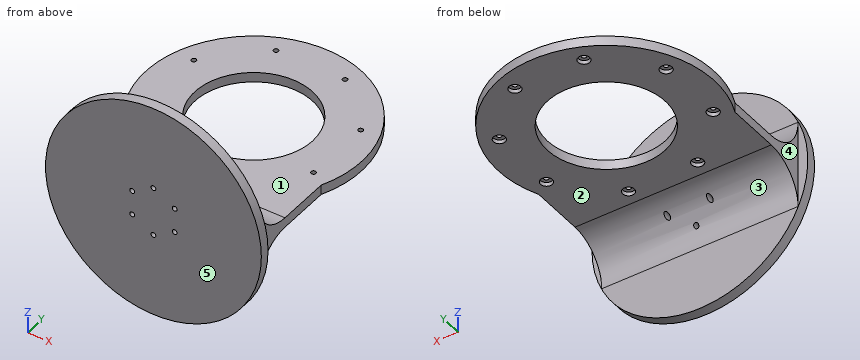
Autodesk Inventor part; units mm, degrees
ref_plane "YZ Plane" through (0, 0, 0) normal (1, 0, 0) x (0, 1, 0)
ref_plane "XZ Plane" through (0, 0, 0) normal (0, 1, 0) x (-1, 0, 0)
ref_plane "XY Plane" through (0, 0, 0) normal (0, 0, 1) x (1, 0, 0)
sketch "スケッチ1" plane through (0, 0, 0) normal (0, 0, 1) x (1, 0, 0)
  circle A0 centre (0, 0) radius 48.5
  circle A1 centre (0, 0) radius 30
  line L0 (-50, 50) -> (50, 50)
  line L1 (50, 50) -> (50, -50)
  line L2 (50, -50) -> (-50, -50)
  line L3 (-50, -50) -> (-50, 50)
  line L4 (-50, -50) -> (50, -50)
  line L5 (50, -50) -> (50, -70)
  line L6 (50, -70) -> (-50, -70)
  line L7 (-50, -70) -> (-50, -50)
  circle A2 centre (0, 0) radius 55
  point P0 (-50, -60)
  point P1 (-50, -22.9129)
  point P2 (50, -22.9129)
  dimension "d0" = 97
  dimension "d3" = 50
  dimension "d4" = 50
  dimension "d5" = 50
  dimension "d6" = 50
  dimension "d126" = 20
  dimension "d127" = 100
  dimension "d128" = 110
  dimension "d129" = 60
extrude "押し出し1" add sketch "スケッチ1" along normal blind 5 contours A0 | A1 | A2 L0 | L0 A2 L1 L2 L3 | L3 A2 | A2 L2 L3 | A2 L1 | L2 A2 L5 L6 L7 | L2 A2 | L1 L2 A2
sketch "スケッチ2" plane through (0, 0, 5) normal (0, 0, 1) x (1, 0, 0)
  circle A0 centre (0, 0) radius 46
  line L0 (0, 0) -> (0, 64.6511)
  line L1 (0, 0) -> (-25.9524, 62.6547)
  line L2 (-50, -22.9129) -> (-50, -70)
  point P0 (-17.6034, 42.4985)
  point P1 (-42.4985, 17.6034)
  point P2 (-42.4985, -17.6034)
  point P3 (-17.6034, -42.4985)
  point P4 (17.6034, -42.4985)
  point P5 (42.4985, -17.6034)
  point P6 (42.4985, 17.6034)
  point P7 (17.6034, 42.4985)
  point P8 (-50, 50)
  point P9 (-50, -50)
  dimension "d7" = 92
  dimension "d8" = 22.5
  dimension "d11" = 360
  dimension "d76" = 50
hole "穴1" at (-17.6034, 42.4985, 5) at (-42.4985, 17.6034, 5) at (-42.4985, -17.6034, 5) at (-17.6034, -42.4985, 5) at (17.6034, -42.4985, 5) at (42.4985, -17.6034, 5) at (42.4985, 17.6034, 5) at (17.6034, 42.4985, 5) direction (0, 0, -1) diameter 2.459 end through all
sketch "スケッチ3" plane through (0, 0, 5) normal (0, 0, 1) x (1, 0, 0)
  circle A0 centre (0, 0) radius 30
  dimension "d20" = 60
extrude "押し出し2" cut sketch "スケッチ3" against normal blind 5
sketch "スケッチ16" plane through (0, 0, 0) normal (0, 0, -1) x (-1, 0, 0)
  circle A0 centre (17.6034, 42.4985) radius 1.2295
  circle A1 centre (0, 0) radius 46
  circle A2 centre (17.6034, 42.4985) radius 3
  circle A3 centre (-17.6034, 42.4985) radius 3
  circle A4 centre (-42.4985, 17.6034) radius 3
  circle A5 centre (-42.4985, -17.6034) radius 3
  circle A6 centre (-17.6034, -42.4985) radius 3
  circle A7 centre (17.6034, -42.4985) radius 3
  circle A8 centre (42.4985, -17.6034) radius 3
  circle A9 centre (42.4985, 17.6034) radius 3
  point P0 (18.7653, 42.0962)
  point P1 (16.4975, 43.0356)
  dimension "d113" = 6
  dimension "d116" = 360
extrude "押し出し12" cut sketch "スケッチ16" against normal blind 2 contours A0 A1 | A0 A1 A2 | A1 A0 | A0 A1 A2 | A3 A1 | A1 A3 | A9 A1 | A1 A9 | A4 A1 | A1 A4 | A8 A1 | A1 A8 | A5 A1 | A1 A5 | A7 A1 | A1 A7 | A6 A1 | A1 A6
sketch "スケッチ19" plane through (-50, -70, 0) normal (0, -1, 0) x (1, 0, 0)
  line L0 (0, 5) -> (100, 5)
  line L1 (0, 5) -> (100, 5)
  line L2 (100, 5) -> (100, -47.5)
  line L3 (100, -47.5) -> (0, -47.5)
  line L4 (0, -47.5) -> (0, 5)
  line L5 (0, -47.5) -> (100, -47.5)
  line L6 (100, -47.5) -> (100, 52.5)
  line L7 (100, 52.5) -> (0, 52.5)
  line L8 (0, 52.5) -> (0, -47.5)
  circle A0 centre (50, 2.5) radius 55
  point P0 (50, 0)
  dimension "d130" = 100
  dimension "d131" = 47.5
  dimension "d132" = 100
  dimension "d136" = 110
  dimension "d137" = 50
  dimension "d138" = 50
extrude "押し出し14" add sketch "スケッチ19" along normal blind 5 contours L8 A0 L7 L6 L0 | L0 L2 A0 L3 L4 | L4 A0 L8 | L6 A0 L2 | L3 A0 | A0 L7
fillet "フィレット6" radius 20 2 edges at (0, -70, 5) (0, -70, 0)
sketch "スケッチ20" plane through (0, -75, 2.5) normal (0, -1, 0) x (1, 0, 0)
  circle A0 centre (0, 0) radius 12.5
  line L0 (-10.8253, -6.25) -> (0, 0)
  line L1 (0, 0) -> (-14.9018, 0)
  point P0 (0, -2.5)
  point P1 (0, -12.5)
  point P2 (10.8253, -6.25)
  point P3 (10.8253, 6.25)
  point P4 (0, 12.5)
  point P5 (-10.8253, 6.25)
  dimension "d139" = 25
  dimension "d140" = 30
  dimension "d143" = 360
hole "穴5" at (-10.8253, -75, -3.75) at (0, -75, -10) at (10.8253, -75, -3.75) at (10.8253, -75, 8.75) at (0, -75, 15) at (-10.8253, -75, 8.75) direction (0, 1, 0) diameter 2.459 end through all
properties part number "legparts_07(five)"
The model under review builds one solid part; all positions refer to its coordinate system, in mm. Face numbers are marked on the shaded views. A direction names the side the tool comes from. Give positions to 0.01 mm unless a question says otherwise; leave off trailing zeros. Write each loop counter-clockwise with the first axis right and the second up, starting at its lowest first coordinate (ties: lowest second). Pieces come first, ordered by that corner, then holes. Notation, with made-up numbers: M 23.5,66.5 L 36.5,66.5 A28 ccw 36.5,102.5 Z; hole C 47.25,85.5 d11. An arc over 180 degrees is marked long. Answer in a Markdown table with one row per item.
Item 1: Add section B-B on x = 35. Give the boundary of the cut face in (y, z), plus the area to 3 significant figures.
Check sheet entries:
| item | result |
|---|---|
| outline | M -75,-39.93 L -70,-39.93 L -70,-20 A20 cw -50,0 L 42.43,0 L 42.43,5 L -50,5 A20 cw -70,25 L -70,44.93 L -75,44.93 Z |
| area | 1,160 mm2 |
Item 2: For line 1 along X through (y, z) = (-68, 8); line 2 along Z through (x, y) = (19.5, -27.5); line 3 along Y through (x, z) = (-27, -24.5), list the stretches that pass through material, from the lowest coordinate up.
Check sheet entries:
| item | result |
|---|---|
| line 1 | -50 to -11.8, -9.85 to 9.85, 11.8 to 50 |
| line 2 | 0 to 5 |
| line 3 | -75 to -70 |
Item 3: Draft analysis for pull direction Y (two halves, no side actions). For the marked faces 3, 4 and 5, state which applies: +Y half, -Y half, draft (parallel to the pull), parting line (faces both ways), or undercut.
Check sheet entries:
| item | result |
|---|---|
| face 3 | +Y half |
| face 4 | undercut |
| face 5 | -Y half |
Item 4: For P1, Ø5, axis at x = -17, y = -41.5, coming from the -Z side; P2, Ø2, axis at x = -10.83, z = 8.75, coming from the +Y side; P3, Ø12, axis at x = -14.5, z = 37.5, coming from the +Y side; P4, Ø3, axis at x = 0, z = -10, coming from the -Y side, all flat-tipped, find the tip position at first contact; note any pin that passes through.
Check sheet entries:
| item | result |
|---|---|
| P1 | z = 0 |
| P2 | through |
| P3 | y = -70 |
| P4 | y = -75 |
Item 5: Add section D-D on y = -61.5. Give the boundary of the cut face in (x, z), plus the area to 3 significant figures.
Check sheet entries:
| item | result |
|---|---|
| outline | M -50,-3.64 L -12.05,-3.64 A1.23 cw -9.6,-3.64 L 9.6,-3.64 A1.23 cw 12.05,-3.64 L 50,-3.64 L 50,8.64 L 12.05,8.64 A1.23 cw 9.6,8.64 L -9.6,8.64 A1.23 cw -12.05,8.64 L -50,8.64 Z |
| area | 1,220 mm2 |
Item 6: Add section C-C on x = 7.5. Give the boundary of the cut face in (y, z), plus the area to 3 significant figures.
Check sheet entries:
| item | result |
|---|---|
| outline | M -75,-51.99 L -70,-51.99 L -70,-20 A20 cw -50,0 L -29.05,0 L -29.05,5 L -50,5 A20 cw -70,25 L -70,56.99 L -75,56.99 Z; M 29.05,0 L 54.49,0 L 54.49,5 L 29.05,5 Z |
| area | 1,050 mm2 |
Item 7: Tool access review of the marked faces 1 and 2: name each direction out of +Z, -Z, +X, -X, +Y, -Y from which nothing blocks a thin tool from reaching the whole face with its end or side.
Check sheet entries:
| item | result |
|---|---|
| face 1 | +Z, +X, -X, +Y |
| face 2 | -Z, +X, -X, +Y |
Item 8: Add section A-A on y = 0. Give the boundary of the cut face in (x, z), plus the area to 3 significant figures.
Check sheet entries:
| item | result |
|---|---|
| outline | M -55,0 L -30,0 L -30,5 L -55,5 Z; M 30,0 L 55,0 L 55,5 L 30,5 Z |
| area | 250 mm2 |
